Could you check a few things on this model? Use its own coordinates, in mm. Coordinates: 2 decimals unless noted, no trailing zeros. Order: outer loops, then holes, each group sorted by start corner. A loop starts at its lowest first (then second) coordinate and runs counter-clockwise, first axis right, second up. Notation, with made-up numbers: (2, 42) - (52, 42) arc R31 ccw to (52, 76) - close; hole circle Ø5 at (63, 86). An arc over 180 degrees is marked (long way). One line per item, written item: value.
from build123d import *

# Parameters (mm, degrees)
EXTRUDE_1_DEPTH     = 3
EXTRUDE_2_DEPTH     = 3
SKETCH_3_R          = 1.6
CUT_EXTRUDE_1_DEPTH = 168.152318263
SKETCH_4_W          = 15
SKETCH_4_H          = 3.5
EXTRUDE_3_DEPTH     = 3
SKETCH_5_R          = 1.6
CUT_EXTRUDE_2_DEPTH = 168.152318263
CHAMFER_1_SIZE      = 0.8
CUT_EXTRUDE_3_DEPTH = 168.054153154
CUT_EXTRUDE_4_DEPTH = 10


with BuildPart() as part:
    # 草图1 → 凸台-拉伸1 (new body)
    with BuildSketch(Plane.XY):
        Polygon((0, 0), (0, 98), (60, 98), (119.771681886, 103.229344565), (128.312944675, 5.602264152), (64.278772405, 0), align=None)
    extrude(amount=EXTRUDE_1_DEPTH)

    # 草图2 → 凸台-拉伸2 (add, through all)
    with BuildSketch(Plane.XY):
        Polygon((119.771681886, 103.229344565), (104.828761414, 101.922008424), (104.523716315, 105.408689867), (119.466636786, 106.716026008), align=None)
        Polygon((79.923893962, 99.743114855), (64.98097349, 98.435778714), (64.675928391, 101.922460157), (79.618848862, 103.229796298), align=None)
        Polygon((128.617989774, 2.115582709), (113.675069303, 0.808246567), (113.370024203, 4.294928011), (128.312944675, 5.602264152), align=None)
        Polygon((88.770201851, -1.370647001), (73.827281379, -2.677983143), (73.52223628, 0.808698301), (88.465156751, 2.116034442), align=None)
    extrude(amount=EXTRUDE_2_DEPTH)

    # 草图3 → 切除-拉伸1 (cut, through all)
    with BuildSketch(Plane.XY):
        with Locations((110.079917707, 99.269583573)):
            Circle(SKETCH_3_R)
        with Locations((100.117970726, 98.398026146)):
            Circle(SKETCH_3_R)
        with Locations((77.20549267, 96.393444063)):
            Circle(SKETCH_3_R)
        with Locations((67.243545689, 95.521886635)):
            Circle(SKETCH_3_R)
        with Locations(Location((118.080814891, 7.818910288, 0), (0, 0, 180))):
            Circle(SKETCH_3_R)
        with Locations(Location((108.11886791, 6.947352861, 0), (0, 0, 180))):
            Circle(SKETCH_3_R)
        with Locations(Location((85.206389854, 4.942770778, 0), (0, 0, 180))):
            Circle(SKETCH_3_R)
        with Locations(Location((75.244442873, 4.07121335, 0), (0, 0, 180))):
            Circle(SKETCH_3_R)
        with BuildLine():
            Line((101.64093838, 101.643110047), (104.828761414, 101.922008424))
            ThreePointArc((104.828761414, 101.922008424), (103.374299086, 100.188647718), (101.64093838, 101.643110047))
        make_face()
        with BuildLine():
            Line((79.923893962, 99.743114855), (83.111716996, 100.022013232))
            ThreePointArc((83.111716996, 100.022013232), (81.657254667, 98.288652526), (79.923893962, 99.743114855))
        make_face()
        with BuildLine():
            Line((61.793150457, 98.156880337), (64.98097349, 98.435778714))
            ThreePointArc((64.98097349, 98.435778714), (63.526511162, 96.702418008), (61.793150457, 98.156880337))
        make_face()
        with BuildLine():
            Line((70.334413246, 0.529799924), (73.52223628, 0.808698301))
            ThreePointArc((73.52223628, 0.808698301), (71.788875574, 2.263160629), (70.334413246, 0.529799924))
        make_face()
        with BuildLine():
            Line((88.465156751, 2.116034442), (91.652979785, 2.394932819))
            ThreePointArc((91.652979785, 2.394932819), (89.91961908, 3.849395147), (88.465156751, 2.116034442))
        make_face()
        with BuildLine():
            Line((110.18220117, 4.016029634), (113.370024203, 4.294928011))
            ThreePointArc((113.370024203, 4.294928011), (111.636663498, 5.749390339), (110.18220117, 4.016029634))
        make_face()
    extrude(amount=CUT_EXTRUDE_1_DEPTH, mode=Mode.SUBTRACT)

    # 草图4 → 凸台-拉伸3 (add, through all)
    with BuildSketch(Plane.XY):
        with Locations((42.5, 99.75)):
            Rectangle(SKETCH_4_W, SKETCH_4_H)
        with Locations((7.5, 99.75)):
            Rectangle(SKETCH_4_W, SKETCH_4_H)
        with Locations((42.5, -1.75)):
            Rectangle(SKETCH_4_W, SKETCH_4_H)
        with Locations((7.5, -1.75)):
            Rectangle(SKETCH_4_W, SKETCH_4_H)
    extrude(amount=EXTRUDE_3_DEPTH)

    # 草图5 → 切除-拉伸2 (cut, through all)
    with BuildSketch(Plane.XY):
        with Locations((3, 94.9)):
            Circle(SKETCH_5_R)
        with Locations((13, 94.9)):
            Circle(SKETCH_5_R)
        with Locations((38, 94.9)):
            Circle(SKETCH_5_R)
        with Locations((48, 94.9)):
            Circle(SKETCH_5_R)
        with Locations(Location((3, 3.1, 0), (0, 0, 180))):
            Circle(SKETCH_5_R)
        with Locations(Location((13, 3.1, 0), (0, 0, 180))):
            Circle(SKETCH_5_R)
        with Locations(Location((48, 3.1, 0), (0, 0, 180))):
            Circle(SKETCH_5_R)
        with Locations(Location((38, 3.1, 0), (0, 0, 180))):
            Circle(SKETCH_5_R)
        with BuildLine():
            Line((15, 98), (18.2, 98))
            ThreePointArc((18.2, 98), (16.6, 96.4), (15, 98))
        make_face()
        with BuildLine():
            Line((31.8, 98), (35, 98))
            ThreePointArc((35, 98), (33.4, 96.4), (31.8, 98))
        make_face()
        with BuildLine():
            Line((50, 98), (53.2, 98))
            ThreePointArc((53.2, 98), (51.6, 96.4), (50, 98))
        make_face()
        with BuildLine():
            Line((50, 0), (53.2, 0))
            ThreePointArc((53.2, 0), (51.6, 1.6), (50, 0))
        make_face()
        with BuildLine():
            Line((31.8, 0), (35, 0))
            ThreePointArc((35, 0), (33.4, 1.6), (31.8, 0))
        make_face()
        with BuildLine():
            Line((15, 0), (18.2, 0))
            ThreePointArc((18.2, 0), (16.6, 1.6), (15, 0))
        make_face()
    extrude(amount=CUT_EXTRUDE_2_DEPTH, mode=Mode.SUBTRACT)

    # 倒角1
    chamfer_1_edges = [part.edges().sort_by_distance(p)[0] for p in [
        (0, 101.5, 1.5),
        (15, 101.5, 1.5),
        (35, -3.5, 1.5),
        (50, -3.5, 1.5),
        (35, 101.5, 1.5),
        (50, 101.5, 1.5),
        (0, -3.5, 1.5),
        (15, -3.5, 1.5),
        (119.466636786, 106.716026008, 1.5),
        (104.523716315, 105.408689867, 1.5),
        (79.618848862, 103.229796298, 1.5),
        (64.675928391, 101.922460157, 1.5),
        (128.617989774, 2.115582709, 1.5),
        (113.675069303, 0.808246567, 1.5),
        (88.770201851, -1.370647001, 1.5),
        (73.827281379, -2.677983143, 1.5),
    ]]
    chamfer(chamfer_1_edges, length=CHAMFER_1_SIZE)

    # 草图6 → 切除-拉伸3 (cut, through all)
    with BuildSketch(Plane.XY):
        with BuildLine():
            Line((88.589794022, 12.165137166), (119.471829663, 14.866965191))
            ThreePointArc((119.471829663, 14.866965191), (121.103967944, 16.001019432), (120.952257678, 17.982669852))
            Line((120.952257678, 17.982669852), (85.230022186, 70.604579281))
            ThreePointArc((85.230022186, 70.604579281), (82.904864414, 71.365551505), (81.582893289, 69.306952531))
            Line((81.582893289, 69.306952531), (86.42309314, 13.983215076))
            ThreePointArc((86.42309314, 13.983215076), (87.129907317, 12.625437676), (88.589794022, 12.165137166))
        make_face()
        with BuildLine():
            Line((119.680582461, 35.428336277), (114.84038261, 90.752073731))
            ThreePointArc((114.84038261, 90.752073731), (114.133568433, 92.109851132), (112.673681728, 92.570151642))
            Line((112.673681728, 92.570151642), (81.791646087, 89.868323617))
            ThreePointArc((81.791646087, 89.868323617), (80.159507806, 88.734269376), (80.311218072, 86.752618956))
            Line((80.311218072, 86.752618956), (116.033453564, 34.130709527))
            ThreePointArc((116.033453564, 34.130709527), (118.358611336, 33.369737303), (119.680582461, 35.428336277))
        make_face()
        with BuildLine():
            Line((51, 81.632404391), (51, 15.56952717))
            ThreePointArc((51, 15.56952717), (51.616973888, 14.124799246), (53.087238775, 13.571430727))
            Line((53.087238775, 13.571430727), (74.244890746, 14.495193762))
            ThreePointArc((74.244890746, 14.495193762), (75.661331586, 15.174598575), (76.150041367, 16.667601691))
            Line((76.150041367, 16.667601691), (70.392282235, 82.479089719))
            ThreePointArc((70.392282235, 82.479089719), (69.718584469, 83.808457848), (68.312654064, 84.302874676))
            Line((68.312654064, 84.302874676), (52.912761225, 83.630500834))
            ThreePointArc((52.912761225, 83.630500834), (51.555272076, 83.015430503), (51, 81.632404391))
        make_face()
    extrude(amount=CUT_EXTRUDE_3_DEPTH, mode=Mode.SUBTRACT)

    # 草图7 → 切除-拉伸4 (cut)
    with BuildSketch(Plane.XY.offset(3)):
        Polygon((35, 98), (35, 0), (27.806316321, -5.327994522), (11.72452964, -8.165956877), (-13.438736579, -4.098210834), (-15.046915247, 45.849926623), (-17.790278858, 82.365042265), (-16.749692661, 87.378775759), (-5.587040729, 104.690346128), (16.549065644, 104.690346128), align=None)
    extrude(amount=-CUT_EXTRUDE_4_DEPTH, mode=Mode.SUBTRACT)


solid = part.part
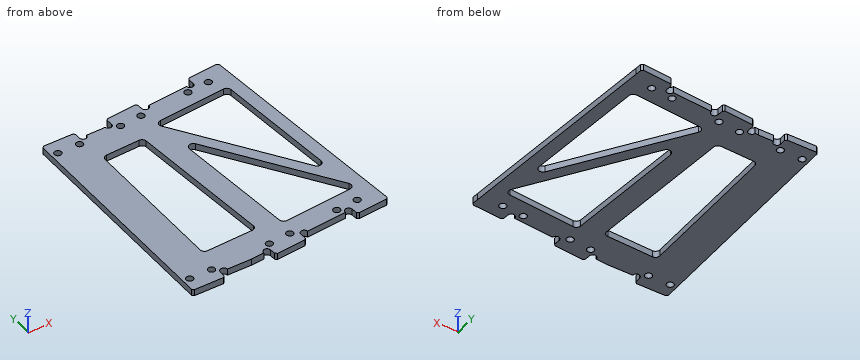
Item 1: I'm going to push flat-ended pins straight in: pin 1 Ø5 at (x, y) = (38, 3.1) entering from +Z; pin 2 Ø1.5 at (y, z) = (41.5, 2) entering from +X; pin 3 Ø0.8 at (y, z) = (99, 1) entering from +X. Where does each tip first touch, or does it pass through?
Conclusion:
pin 1: z = 3
pin 2: x = 125.24
pin 3: x = 120.18
Item 2: If I drill on probe 1 along Y at (x, z) = (48, 0.65); probe 2 along X at (y, z) = (70.5, 0.2); probe 3 along X at (y, z) = (38.5, 0.3), over which ranges is the centre line in solid material (lowest first)?
Conclusion:
probe 1: -3.5 to 1.5, 4.7 to 93.3, 96.5 to 101.5
probe 2: 35 to 51, 71.44 to 81.85, 85.3 to 91.34, 116.61 to 122.64
probe 3: 35 to 51, 74.24 to 84.28, 107.02 to 113.07, 119.41 to 125.43
Item 3: I want a section at B-B on y = 63. Please give me the cut outline in (x, z), then the cut area to 3 significant figures.
Conclusion:
outline: (35, 0) - (51, 0) - (51, 3) - (35, 3) - close; (72.1, 0) - (82.13, 0) - (82.13, 3) - (72.1, 3) - close; (90.39, 0) - (96.44, 0) - (96.44, 3) - (90.39, 3) - close; (117.27, 0) - (123.29, 0) - (123.29, 3) - (117.27, 3) - close
area: 114 mm²
Item 4: I want a section at A-A on x = 48. Please give me the cut outline in (y, z), then the cut area to 3 significant figures.
Conclusion:
outline: (-3.5, 0) - (1.5, 0) - (1.5, 3) - (-3.5, 3) - close; (4.7, 0) - (93.3, 0) - (93.3, 3) - (4.7, 3) - close; (96.5, 0) - (101.5, 0) - (101.5, 3) - (96.5, 3) - close
area: 296 mm²
Item 5: I want a section at C-C on z = 2.15. Give the number of separate pieces and of enclosed holes in the cut face, then the cut area to 3 significant figures.
Conclusion:
separate pieces: 1
enclosed holes: 15
area: 5,030 mm²
